Work out the finished part from the listing and answer in its coordinate system (mm). Face numbers are marked on the shaded views. A direction names the side the tool comes from. Round coordinates to 2 decimals unless told otherwise and drop trailing zeros. Order: outer loops, then holes, each group sorted by start corner. A loop starts at its lowest first (then second) coordinate and runs counter-clockwise, first axis right, second up. Notation, with made-up numbers: (50.25, 17) - (101.25, 17) arc R24 ccw to (101.25, 56) - close; hole circle Ø7 at (12.5, 67). An arc over 180 degrees is marked (long way). Put each result on its own line as item: value.
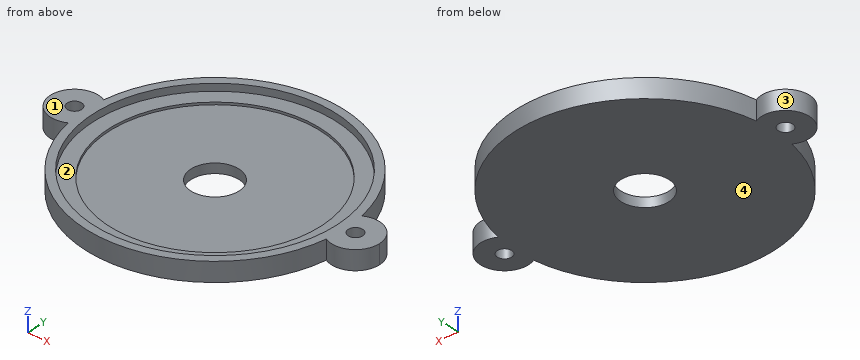
```python
from build123d import *

# Parameters (mm, degrees)
F0_R     = 1.5
F1_DEPTH = 4
F2_DEPTH = 2
F3_R     = 27
F3_R_2   = 22.1
F4_DEPTH = 0.5
F5_R     = 25.3
F6_DEPTH = 1.5
F7_R     = 5
F8_DEPTH = 25


with BuildPart() as f1:
    # F0 (on Top) → F1 (new body)
    with BuildSketch(Plane.XY):
        with BuildLine():
            ThreePointArc((-26.6379310345, -4.4068844099), (-27, 0), (-26.6379310345, 4.4068844099))
            ThreePointArc((-26.6379310345, 4.4068844099), (-34, 0), (-26.6379310345, -4.4068844099))
        make_face()
        with Locations((-29, 0)):
            Circle(F0_R, mode=Mode.SUBTRACT)
    extrude(amount=F1_DEPTH)



with BuildPart() as f1b:
    # F0 (on Top) → F1, piece 2 (new body)
    with BuildSketch(Plane.XY):
        with BuildLine():
            ThreePointArc((26.6379310345, 4.4068844099), (26.9093305187, 2.21086658), (27, 0))
            ThreePointArc((27, 0), (26.9093305187, -2.21086658), (26.6379310345, -4.4068844099))
            ThreePointArc((26.6379310345, -4.4068844099), (31.5680396388, -4.2901249881), (34, 0))
            ThreePointArc((34, 0), (31.5680396388, 4.2901249881), (26.6379310345, 4.4068844099))
        make_face()
        with Locations((29, 0)):
            Circle(F0_R, mode=Mode.SUBTRACT)
    extrude(amount=F1_DEPTH)


with BuildPart() as f2:
    # F0 (on Top) → F2 (new body)
    with BuildSketch(Plane.XY):
        with BuildLine():
            ThreePointArc((-24, 0), (-24.7098750119, 2.5680396388), (-26.6379310345, 4.4068844099))
            ThreePointArc((-26.6379310345, 4.4068844099), (-27, 0), (-26.6379310345, -4.4068844099))
            ThreePointArc((-26.6379310345, -4.4068844099), (-24.7098750119, -2.5680396388), (-24, 0))
        make_face()
        with BuildLine():
            ThreePointArc((26.6379310345, -4.4068844099), (26.9093305187, -2.21086658), (27, 0))
            ThreePointArc((27, 0), (26.9093305187, 2.21086658), (26.6379310345, 4.4068844099))
            ThreePointArc((26.6379310345, 4.4068844099), (24, 0), (26.6379310345, -4.4068844099))
        make_face()
        with BuildLine():
            ThreePointArc((26.6379310345, -4.4068844099), (24, 0), (26.6379310345, 4.4068844099))
            ThreePointArc((26.6379310345, 4.4068844099), (0, 27), (-26.6379310345, 4.4068844099))
            ThreePointArc((-26.6379310345, 4.4068844099), (-24.7098750119, 2.5680396388), (-24, 0))
            ThreePointArc((-24, 0), (-24.7098750119, -2.5680396388), (-26.6379310345, -4.4068844099))
            ThreePointArc((-26.6379310345, -4.4068844099), (0, -27), (26.6379310345, -4.4068844099))
        make_face()
    extrude(amount=F2_DEPTH)


with BuildPart() as f1_1:
    add(f1.part)

    add(f1b.part)  # F4 merges F1b

    add(f2.part)  # F4 merges F2
    # F3 (on face) → F4 (join)
    with BuildSketch(Plane.XY.offset(2)):
        Circle(F3_R)
        Circle(F3_R_2, mode=Mode.SUBTRACT)
    extrude(amount=F4_DEPTH)

    # F5 (on face) → F6 (join)
    with BuildSketch(Plane.XY.offset(2.5)):
        with BuildLine():
            ThreePointArc((26.6379310345, -4.4068844099), (27, 0), (26.6379310345, 4.4068844099))
            ThreePointArc((26.6379310345, 4.4068844099), (0, 27), (-26.6379310345, 4.4068844099))
            ThreePointArc((-26.6379310345, 4.4068844099), (-27, 0), (-26.6379310345, -4.4068844099))
            ThreePointArc((-26.6379310345, -4.4068844099), (0, -27), (26.6379310345, -4.4068844099))
        make_face()
        Circle(F5_R, mode=Mode.SUBTRACT)
    extrude(amount=F6_DEPTH)

    # F7 (on face) → F8 (cut)
    with BuildSketch(Plane.XY.offset(2)):
        Circle(F7_R)
    extrude(amount=-F8_DEPTH, mode=Mode.SUBTRACT)


solid = f1_1.part
```
1) Straight lines are drawn through the part: L1, parallel to X at y = -4.5, z = 1.7; L2, parallel to Z at x = 11.5, y = -20.5; L3, parallel to Z at x = 5, y = 13.5. For each, find the intervals that lie inside material, in ascending order. Write a range as from..to.
Findings below:
L1: x = -31.18..-26.82, -26.62..-2.18, 2.18..26.62, 26.82..31.18
L2: z = 0..2.5
L3: z = 0..2
2) A cutting plane is placed at D-D on x = 29. Write down the section's boundary in (y, z).
Findings below:
outline: (-5, 0) - (-1.5, 0) - (-1.5, 4) - (-5, 4) - close; (1.5, 0) - (5, 0) - (5, 4) - (1.5, 4) - close
3) For a pull along X with two mould halves and no side action, classify the marked faces 3 and 4 as pulls with the +X half, pulls with the -X half, needs draft (parallel to the pull), parting line crosses it, or undercut.
Findings below:
face 3: undercut
face 4: needs draft
4) A cutting plane is placed at B-B on z = 1.35. Write down the section's boundary in (x, y).
Findings below:
outline: (-26.64, -4.41) arc R27 ccw to (26.64, -4.41) arc R5 ccw (long way) to (26.64, 4.41) arc R27 ccw to (-26.64, 4.41) arc R5 ccw (long way) to start; hole circle Ø3 at (-29, 0); hole circle Ø10 at (0, 0); hole circle Ø3 at (29, 0)
5) For the marked faces 1 and 2, determine the directions among +Z, -Z, +X, -X, +Y, -Y from which every point of the face is accessible in a straight line to the end or side of a thin tool.
Findings below:
face 1: +Z, +X, -X, +Y, -Y
face 2: +Z
6) A cutting plane is placed at C-C on y = -14.5. Write down the section's boundary in (x, z).
Findings below:
outline: (-22.78, 0) - (22.78, 0) - (22.78, 4) - (20.73, 4) - (20.73, 2.5) - (16.68, 2.5) - (16.68, 2) - (-16.68, 2) - (-16.68, 2.5) - (-20.73, 2.5) - (-20.73, 4) - (-22.78, 4) - close
7) Given pin 1 Ø1 at (y, z) = (19, 2.5) entering from -X; pin 2 Ø2 at (x, z) = (22.5, 1.5) entering from +Y; pin 3 Ø16 at (x, y) = (0, 0) entering from +Z, each flat-ended and moving along its own axis, determine where each tip first touches the part or whether it passes through.
Findings below:
pin 1: stops at x = -19.67
pin 2: stops at y = 16.33
pin 3: stops at z = 2
8) A cutting plane is placed at A-A on x = 0. Write down the section's boundary in (y, z), then the cut area to 3 significant figures.
Findings below:
outline: (-27, 0) - (-5, 0) - (-5, 2) - (-22.1, 2) - (-22.1, 2.5) - (-25.3, 2.5) - (-25.3, 4) - (-27, 4) - close; (5, 0) - (27, 0) - (27, 4) - (25.3, 4) - (25.3, 2.5) - (22.1, 2.5) - (22.1, 2) - (5, 2) - close
area: 98.0 mm2
